Could you check a few things on this drawing? It's one solid part, dimensions in mm from its lowest x, y, z. Coordinates: 2 decimals unless noted, no trailing zeros. Loops run counter-clockwise (first coordinate to the right, second up) from the corner with the lowest first, then second, coordinate; pieces in that order, holes last. Notation, with made-up numbers: (-4, -37.75) -> (14, -37.75) arc R28 ccw to (14, -19.75) -> close; hole circle Ø2 at (18, 48). An arc over 180 degrees is marked (long way). One line per question, with ' | ' between items.
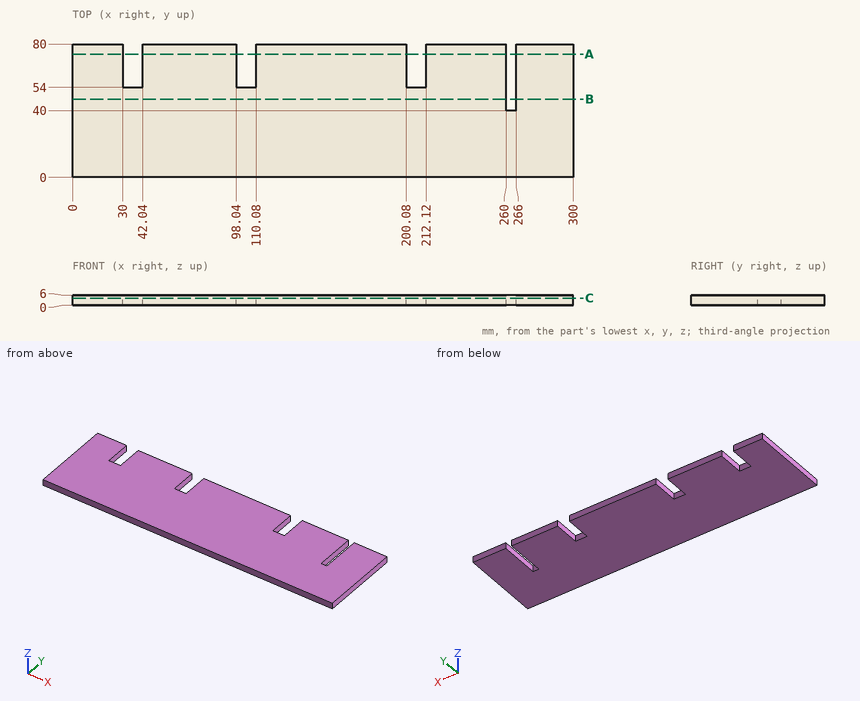
1) If we section it at B-B on y = 47: Please give me the cut outline in (x, z).
Data:
outline: (0, 0) -> (260, 0) -> (260, 6) -> (0, 6) -> close; (266, 0) -> (300, 0) -> (300, 6) -> (266, 6) -> close
2) If we section it at A-A on y = 74: Please give me the cut outline in (x, z).
Data:
outline: (0, 0) -> (30, 0) -> (30, 6) -> (0, 6) -> close; (42.04, 0) -> (98.04, 0) -> (98.04, 6) -> (42.04, 6) -> close; (110.08, 0) -> (200.08, 0) -> (200.08, 6) -> (110.08, 6) -> close; (212.12, 0) -> (260, 0) -> (260, 6) -> (212.12, 6) -> close; (266, 0) -> (300, 0) -> (300, 6) -> (266, 6) -> close
3) I'm going to push a flat-ended pin straight in: pin 1 Ø3 at (x, z) = (37.5, 1.5) entering from +Y. Where does the tip first touch, or does it pass through?
Data:
pin 1: y = 54
4) I need wall thicknesses on line 1 along X through (y, z) = (65, 4.75); line 2 along X through (y, z) = (53, 2.3); line 3 along Y through (x, z) = (105.5, 1.3). Which ranges of each line are inside material? Lowest first, please. Write a range as from..to.
Data:
line 1: 0..30, 42.04..98.04, 110.08..200.08, 212.12..260, 266..300 | line 2: 0..260, 266..300 | line 3: 0..54
5) If we section it at C-C on z = 4.35: Please give me the cut outline in (x, y).
Data:
outline: (0, 0) -> (300, 0) -> (300, 80) -> (266, 80) -> (266, 40) -> (260, 40) -> (260, 80) -> (212.12, 80) -> (212.12, 54) -> (200.08, 54) -> (200.08, 80) -> (110.08, 80) -> (110.08, 54) -> (98.04, 54) -> (98.04, 80) -> (42.04, 80) -> (42.04, 54) -> (30, 54) -> (30, 80) -> (0, 80) -> close
